Model file for the job. Use its own axes, mm. Give positions to 0.01 mm unless a question says otherwise; leave off trailing zeros. Loops run counter-clockwise (first coordinate to the right, second up) from the corner with the lowest first, then second, coordinate; pieces in that order, holes last. Notation, with made-up numbers: (72, -3.75) - (78, -3.75) arc R20 ccw to (78, 15.25) - close; hole circle Ø6 at (58.5, 43). An arc over 180 degrees is marked (long way). Use a Markdown table: item, result.
from build123d import *

# Parameters (mm, degrees)
SKETCH_1_R          = 18
EXTRUDE_1_DEPTH     = 9
SKETCH_2_R          = 1.525
CUT_EXTRUDE_1_DEPTH = 10
SKETCH_3_R          = 10.5
CUT_EXTRUDE_2_DEPTH = 10


with BuildPart() as part:
    # 草图1 → 凸台-拉伸1 (new body)
    with BuildSketch(Plane(origin=(0, 0, 0), x_dir=(1, 0, 0), z_dir=(0, 1, 0))):
        Circle(SKETCH_1_R)
    extrude(amount=EXTRUDE_1_DEPTH)

    # 草图2 → 切除-拉伸1 (cut, through all)
    with BuildSketch(Plane(origin=(0, 9, 0), x_dir=(1, 0, 0), z_dir=(0, 1, 0))):
        with Locations((13.5, 0)):
            Circle(SKETCH_2_R)
        with Locations((6.75, -11.691342951)):
            Circle(SKETCH_2_R)
        with Locations((-6.75, -11.691342951)):
            Circle(SKETCH_2_R)
        with Locations((-13.5, 0)):
            Circle(SKETCH_2_R)
        with Locations((-6.75, 11.691342951)):
            Circle(SKETCH_2_R)
        with Locations((6.75, 11.691342951)):
            Circle(SKETCH_2_R)
    extrude(amount=-CUT_EXTRUDE_1_DEPTH, mode=Mode.SUBTRACT)

    # 草图3 → 切除-拉伸2 (cut, through all)
    with BuildSketch(Plane(origin=(0, 9, 0), x_dir=(1, 0, 0), z_dir=(0, 1, 0))):
        Circle(SKETCH_3_R)
    extrude(amount=-CUT_EXTRUDE_2_DEPTH, mode=Mode.SUBTRACT)


solid = part.part
(1) Slice it at D-D, the plane y = 8.25. Write the cut outline in (x, z) (3 decimals).
Computed:
| item | result |
|---|---|
| outline | circle Ø36 at (0, 0); hole circle Ø3.05 at (-13.5, 0); hole circle Ø21 at (0, 0); hole circle Ø3.05 at (-6.75, -11.691); hole circle Ø3.05 at (-6.75, 11.691); hole circle Ø3.05 at (6.75, -11.691); hole circle Ø3.05 at (6.75, 11.691); hole circle Ø3.05 at (13.5, 0) |
(2) Drill centre lines: probe 1 along X at (y, z) = (4, 0) (3 decimals); probe 2 along Z at (x, y) = (6.75, 3); probe 3 along X at (y, z) = (1.25, 0.5). Where is each one in solid material? Low to high. Write a range as [from, to].
Computed:
| item | result |
|---|---|
| probe 1 | [-18, -15.025], [-11.975, -10.5], [10.5, 11.975], [15.025, 18] |
| probe 2 | [-16.69, -13.22], [-10.17, -8.04], [8.04, 10.17], [13.22, 16.69] |
| probe 3 | [-17.99, -14.94], [-12.06, -10.49], [10.49, 12.06], [14.94, 17.99] |
(3) Slice it at C-C, the plane x = 6.75. Write the cut outline in (y, z).
Computed:
| item | result |
|---|---|
| outline | (0, -16.69) - (9, -16.69) - (9, -13.22) - (0, -13.22) - close; (0, -10.17) - (9, -10.17) - (9, -8.04) - (0, -8.04) - close; (0, 8.04) - (9, 8.04) - (9, 10.17) - (0, 10.17) - close; (0, 13.22) - (9, 13.22) - (9, 16.69) - (0, 16.69) - close |
(4) Pin check, flat tips, straight feed: P1, Ø2, axis at y = 7, z = 8, coming from the -X side; P2, Ø12, axis at x = -4, z = -0.5, coming from the +Y side; P3, Ø1, axis at y = 5.5, z = 8, coming from the -X side. Stop position of each tip, or through.
Computed:
| item | result |
|---|---|
| P1 | x = -16.58 |
| P2 | through |
| P3 | x = -16.36 |
(5) Slice it at A-A, the plane x = 0. Write the cut outline in (y, z), plus the area to 3 significant figures.
Computed:
| item | result |
|---|---|
| outline | (0, -18) - (9, -18) - (9, -10.5) - (0, -10.5) - close; (0, 10.5) - (9, 10.5) - (9, 18) - (0, 18) - close |
| area | 135 mm² |
(6) Slice it at B-B, the plane z = 9. Write the cut outline in (x, y), plus the area to 3 significant figures.
Computed:
| item | result |
|---|---|
| outline | (-15.59, 0) - (-5.41, 0) - (-5.41, 9) - (-15.59, 9) - close; (5.41, 0) - (15.59, 0) - (15.59, 9) - (5.41, 9) - close |
| area | 183 mm² |
(7) Mould opens along Z. For faces 1 (the flat face through (8, 0, 8)), 2 (the cylindrical face through (-6.949, 4.563, -13.203)), 3 (the cylindrical face through (-2.343, 4.437, -17.847)), 4 (the cylindrical face through (14.9, 4.6, 0.6)) say: pulls with the +Z half, pulls with the -Z half, needs draft (parallel to the pull), parting line crosses it, or undercut.
Computed:
| item | result |
|---|---|
| face 1 | needs draft |
| face 2 | undercut |
| face 3 | parting line crosses it |
| face 4 | undercut |
